from build123d import *

# Parameters (mm, degrees)
SKETCH1_W                      = 464.2
SKETCH1_H                      = 468
BASE_FLANGE1_DEPTH             = 3.2
EDGE_FLANGE1_STRIP_W           = 14.8
EDGE_FLANGE1_STRIP_H           = 3.2
EDGE_FLANGE1_STRIP_CUT_DEPTH   = 464.2
EDGE_FLANGE1_DEPTH             = 464.2
EDGE_FLANGE2_STRIP_W           = 14.8
EDGE_FLANGE2_STRIP_H           = 3.2
EDGE_FLANGE2_STRIP_CUT_DEPTH   = 464.2
EDGE_FLANGE2_DEPTH             = 464.2
SKETCH12_W                     = 2.3
SKETCH12_H                     = 459.6
SKETCH12_H_2                   = 462.8
SKETCH12_H_3                   = 463.8
BOSS_EXTRUDE1_DEPTH            = 200
EDGE_FLANGE3_STRIP_W           = 14.8
EDGE_FLANGE3_STRIP_H           = 3.2
EDGE_FLANGE3_STRIP_CUT_DEPTH   = 459.6
EDGE_FLANGE3_STRIP_2_W         = 14.8
EDGE_FLANGE3_STRIP_2_H         = 3.2
EDGE_FLANGE3_STRIP_CUT_2_DEPTH = 459.6
EDGE_FLANGE3_DEPTH             = 459.6
EDGE_FLANGE3_BEND_DEPTH        = 459.6


# Sheet-metal steps are written as plain solids
with BuildPart() as part:
    # Sketch1 → Base-Flange1 (new body)
    with BuildSketch(Plane(origin=(0, 0, 0), x_dir=(1, 0, 0), z_dir=(0, 1, 0))):
        with Locations((23.545430809, -47.580156658)):
            Rectangle(SKETCH1_W, SKETCH1_H)
    extrude(amount=-BASE_FLANGE1_DEPTH)

    # Edge-Flange1 strip (across the edge) → Edge-Flange1 strip cut (cut)
    with BuildSketch(Plane(origin=(255.645430809, 0, -186.419843342), x_dir=(0, 0, 1), z_dir=(-1, 0, 0))):
        with Locations((-3.2, -1.6)):
            Rectangle(EDGE_FLANGE1_STRIP_W, EDGE_FLANGE1_STRIP_H)
    extrude(amount=EDGE_FLANGE1_STRIP_CUT_DEPTH, mode=Mode.SUBTRACT)

    # Edge-Flange1 section (across the edge) → Edge-Flange1 (add)
    with BuildSketch(Plane(origin=(255.645430809, 0, -186.419843342), x_dir=(0, 0, 1), z_dir=(-1, 0, 0))):
        with BuildLine():
            Line((0, 1), (0, 201.8))
            Line((0, 201.8), (3.2, 201.8))
            Line((3.2, 201.8), (3.2, 1))
            ThreePointArc((3.2, 1), (3.492893219, 0.292893219), (4.2, 0))
            Line((4.2, 0), (4.2, -3.2))
            ThreePointArc((4.2, -3.2), (1.230151519, -1.969848481), (0, 1))
        make_face()
    extrude(amount=EDGE_FLANGE1_DEPTH)

    # Edge-Flange2 strip (across the edge) → Edge-Flange2 strip cut (cut)
    with BuildSketch(Plane(origin=(-208.554569191, 0, 281.580156658), x_dir=(0, 0, -1), z_dir=(1, 0, 0))):
        with Locations((-3.2, -1.6)):
            Rectangle(EDGE_FLANGE2_STRIP_W, EDGE_FLANGE2_STRIP_H)
    extrude(amount=EDGE_FLANGE2_STRIP_CUT_DEPTH, mode=Mode.SUBTRACT)

    # Edge-Flange2 section (across the edge) → Edge-Flange2 (add)
    with BuildSketch(Plane(origin=(-208.554569191, 0, 281.580156658), x_dir=(0, 0, -1), z_dir=(1, 0, 0))):
        with BuildLine():
            Line((0, 1), (0, 201.8))
            Line((0, 201.8), (3.2, 201.8))
            Line((3.2, 201.8), (3.2, 1))
            ThreePointArc((3.2, 1), (3.492893219, 0.292893219), (4.2, 0))
            Line((4.2, 0), (4.2, -3.2))
            ThreePointArc((4.2, -3.2), (1.230151519, -1.969848481), (0, 1))
        make_face()
    extrude(amount=EDGE_FLANGE2_DEPTH)

    # Sketch12 → Boss-Extrude1 (add)
    with BuildSketch(Plane(origin=(0, 0, 0), x_dir=(1, 0, 0), z_dir=(0, 1, 0))):
        with Locations((163.495430809, -47.580156658)):
            Rectangle(SKETCH12_W, SKETCH12_H)
        with Locations((70.195430809, -49.180156658)):
            Rectangle(SKETCH12_W, SKETCH12_H_2)
        with Locations((-23.104569191, -49.680156658)):
            Rectangle(SKETCH12_W, SKETCH12_H_3)
        with Locations((-116.404569191, -49.680156658)):
            Rectangle(SKETCH12_W, SKETCH12_H_3)
    extrude(amount=BOSS_EXTRUDE1_DEPTH)

    # Edge-Flange3 strip (across the edge) → Edge-Flange3 strip cut (cut)
    with BuildSketch(Plane(origin=(255.645430809, 0, 277.380156658), x_dir=(-1, 0, 0), z_dir=(0, 0, -1))):
        with Locations((-3.2, -1.6)):
            Rectangle(EDGE_FLANGE3_STRIP_W, EDGE_FLANGE3_STRIP_H)
    extrude(amount=EDGE_FLANGE3_STRIP_CUT_DEPTH, mode=Mode.SUBTRACT)

    # Edge-Flange3 strip 2 (across the edge) → Edge-Flange3 strip cut 2 (cut)
    with BuildSketch(Plane(origin=(-208.554569191, 0, -182.219843342), x_dir=(1, 0, 0), z_dir=(0, 0, 1))):
        with Locations((-3.2, -1.6)):
            Rectangle(EDGE_FLANGE3_STRIP_2_W, EDGE_FLANGE3_STRIP_2_H)
    extrude(amount=EDGE_FLANGE3_STRIP_CUT_2_DEPTH, mode=Mode.SUBTRACT)

    # Edge-Flange3 section (across the edge) → Edge-Flange3 (add)
    with BuildSketch(Plane(origin=(255.645430809, 0, 277.380156658), x_dir=(-1, 0, 0), z_dir=(0, 0, -1))):
        with BuildLine():
            Line((0, 1), (0, 201.8))
            Line((0, 201.8), (3.2, 201.8))
            Line((3.2, 201.8), (3.2, 1))
            ThreePointArc((3.2, 1), (3.492893219, 0.292893219), (4.2, 0))
            Line((4.2, 0), (4.2, -3.2))
            ThreePointArc((4.2, -3.2), (1.230151519, -1.969848481), (0, 1))
        make_face()
    extrude(amount=EDGE_FLANGE3_DEPTH)

    # Edge-Flange3 section 2 (across the edge) → Edge-Flange3 bend (add)
    with BuildSketch(Plane(origin=(-208.554569191, 0, -182.219843342), x_dir=(1, 0, 0), z_dir=(0, 0, 1))):
        with BuildLine():
            Line((0, 1), (0, 201.8))
            Line((0, 201.8), (3.2, 201.8))
            Line((3.2, 201.8), (3.2, 1))
            ThreePointArc((3.2, 1), (3.492893219, 0.292893219), (4.2, 0))
            Line((4.2, 0), (4.2, -3.2))
            ThreePointArc((4.2, -3.2), (1.230151519, -1.969848481), (0, 1))
        make_face()
    extrude(amount=EDGE_FLANGE3_BEND_DEPTH)


solid = part.part
Can you work these out from the model? Positions are in its coordinate system, mm. A direction names the side the tool comes from. Coordinates: 2 decimals unless noted, no trailing zeros. Write each loop counter-clockwise with the first axis right and the second up, starting at its lowest first coordinate (ties: lowest second). Pieces come first, ordered by that corner, then holes. Notation, with made-up numbers: (-1, 78.25) -> (43, 78.25) arc R24 cw to (43, 112.25) -> close; hole circle Ø9 at (-32.5, -31). An arc over 180 degrees is marked (long way). Write item = value, one per line.
(1) Imagine slicing it at C-C (x = 112). Please give me the cut outline in (y, z), and give its area (3 significant figures).
Verdict:
outline = (-3.2, -182.22) arc R4.2 ccw to (1, -186.42) -> (201.8, -186.42) -> (201.8, -183.22) -> (1, -183.22) arc R1 cw to (0, -182.22) -> (0, 277.38) arc R1 cw to (1, 278.38) -> (201.8, 278.38) -> (201.8, 281.58) -> (1, 281.58) arc R4.2 ccw to (-3.2, 277.38) -> close
area = 2,780 mm^2
(2) Thinking about a two-plate mould opening in Z: for faces 1 (the face through (-117.555, 99, 51)), 2 (the face through (20, 99, 281.58)), 3 (the face through (-115.255, 99, 51)), 4 (the face through (-208.555, 100, 44)), which applies, +Z half, -Z half, draft (parallel to the pull), parting line (faces both ways), or undercut?
Verdict:
face_1 = undercut
face_2 = +Z half
face_3 = undercut
face_4 = draft
(3) For pin 1 (12 mm diameter, centred on x = 134.5, z = 115, fed in from +Y); pin 2 (3.5 mm diameter, centred on x = 253.5, y = -1.5, fed in from +Z); pin 3 (1.8 mm diameter, centred on x = -23.5, z = 96.5, fed in from +Y), each with a flat end and sliding along its axis, tell me the tip position at first contact or that it passes through.
Verdict:
pin_1 = 0
pin_2 = 281.51
pin_3 = 200
(4) Imagine slicing it at A-A (y = 87). State how many separate pieces and enclosed holes the cut face has, and give its area (3 significant figures).
Verdict:
separate_pieces = 5
enclosed_holes = 0
area = 10,100 mm^2
(5) If I drill on probe 1 along X at (y, z) = (185.5, -154.5); probe 2 along Z at (x, y) = (-96, 112); probe 3 along Y at (x, z) = (-147.5, -133.5), over which ranges is the centre line in solid material (lowest first)?
Verdict:
probe_1 = -208.55 to -205.35, -117.55 to -115.25, -24.25 to -21.95, 69.05 to 71.35, 162.35 to 164.65, 252.45 to 255.65
probe_2 = -186.42 to -183.22, 278.38 to 281.58
probe_3 = -3.2 to 0
(6) On a 3-axis mill with a long thin cutter (end or side, diameter ignored), from which of +Z, -Z, +X, -X, +Y, -Y can I reach the whole of each face in a straight line? I mean faces 5 (the face through (20, -3.2, 44)), 6 (the face through (207, 0, 44)), 7 (the face through (27, 103, -183.22)). Say none if no direction works.
Verdict:
face_5 = +Z, -Z, +X, -X, -Y
face_6 = +Y
face_7 = +X, -X, +Y
(7) Imagine slicing it at B-B (z = 190). Please give me the cut outline in (x, y).
Verdict:
outline = (-208.55, 1) arc R4.2 ccw to (-204.35, -3.2) -> (251.45, -3.2) arc R4.2 ccw to (255.65, 1) -> (255.65, 201.8) -> (252.45, 201.8) -> (252.45, 1) arc R1 cw to (251.45, 0) -> (164.65, 0) -> (164.65, 200) -> (162.35, 200) -> (162.35, 0) -> (71.35, 0) -> (71.35, 200) -> (69.05, 200) -> (69.05, 0) -> (-21.95, 0) -> (-21.95, 200) -> (-24.25, 200) -> (-24.25, 0) -> (-115.25, 0) -> (-115.25, 200) -> (-117.55, 200) -> (-117.55, 0) -> (-204.35, 0) arc R1 cw to (-205.35, 1) -> (-205.35, 201.8) -> (-208.55, 201.8) -> close
